Design review of the part built by this model. Coordinates are the model's own, in mm. A direction names the side the tool comes from. Coordinates: 2 decimals unless noted, no trailing zeros. Loops run counter-clockwise (first coordinate to the right, second up) from the corner with the lowest first, then second, coordinate; pieces in that order, holes last. Notation, with made-up numbers: (62.5, 24.25) -> (97.5, 24.25) arc R20 cw to (97.5, 41.25) -> close; hole circle Ø4 at (19, 31.5). An arc over 180 degrees is marked (long way). One line per item, written item: value. Start each with the question number.
1. Insertion check: pin 1 (8.5 mm diameter, centred on y = 10.75, z = -22.81, fed in from +X); pin 2 (5 mm diameter, centred on x = -26, y = 7.5, fed in from -Z); pin 3 (0.8 mm diameter, centred on x = 35, y = -48, fed in from -Z); pin 4 (0.8 mm diameter, centred on x = 35, y = 10.5, fed in from +Z). Each pin has a flat end and moves straight along its axis. Give the tip position at first contact, or say it passes through.
2. Add section B-B on z = -6. Write out the cut boundary in (x, y), plus the area to 3 significant figures.
3. Add section C-C on y = 41. Write out the cut boundary in (x, z), plus the area to 3 significant figures.
4. Add section A-A on x = 25. Write out the cut boundary in (y, z).
5. Draft analysis for pull direction X (two halves, no side actions). For faces 4 (the flat face through (34.5, -1, -53)), 5 (the flat face through (35.5, -1, -53)), 6 (the cylindrical face through (-35.007, -60.12, -8.277)), state which applies: pulls with the +X half, pulls with the -X half, needs draft (parallel to the pull), parting line crosses it, or undercut.
6. For probe 1 along X at (y, z) = (-39.5, -15); probe 2 along X at (y, z) = (-25, -29); probe 3 along Z at (x, y) = (-17, -59), list the stretches that pass through material, from the lowest coordinate up.
7. Machinability: for faces 1 (the cylindrical face through (-35.007, -59.896, -40.095)), 2 (the flat face through (-28, -5, -1)), 3 (the cylindrical face through (-35.007, 11.24, -26.555)), which of the approach directions +Z, -Z, +X, -X, +Y, -Y give a long, thin tool a straight path to every point of the face, cutting with its end or side? Answer none if there is none.
8. Add section D-D on y = 25. Write out the cut boundary in (x, z), plus the area to 3 significant figures.
```python
from build123d import *

# Parameters (mm, degrees)
BASE_FLANGE1_START             = -1
BASE_FLANGE1_OUTLINE_W         = 71
BASE_FLANGE1_OUTLINE_H         = 146.600550732
BASE_FLANGE1_DEPTH             = 1
EDGE_FLANGE1_STRIP_W           = 5.4732
EDGE_FLANGE1_STRIP_H           = 1
EDGE_FLANGE1_STRIP_CUT_DEPTH   = 146.600550732
EDGE_FLANGE1_STRIP_2_W         = 5.4732
EDGE_FLANGE1_STRIP_2_H         = 1
EDGE_FLANGE1_STRIP_CUT_2_DEPTH = 146.600550732
EDGE_FLANGE1_DEPTH             = 146.600550732
EDGE_FLANGE1_PROFILE_W         = 56.545302405
EDGE_FLANGE1_PROFILE_H         = 38.800406569
EDGE_FLANGE1_FLAT_DEPTH        = 1
EDGE_FLANGE1_BEND_DEPTH        = 146.600550732
EDGE_FLANGE1_PROFILE_2_W       = 146.600550732
EDGE_FLANGE1_PROFILE_2_H       = 72.095455735
EDGE_FLANGE1_PROFILE_2_R       = 3.775798506
EDGE_FLANGE1_PROFILE_2_R_2     = 3.613625218
EDGE_FLANGE1_FLAT_2_DEPTH      = 1


# Read off the part's stored shape, not the designer's step: Base-Flange1
# Sheet-metal steps are written as plain solids
with BuildPart() as part:
    # Base-Flange1 outline → Base-Flange1 (new body)
    with BuildSketch(Plane.XY.offset(BASE_FLANGE1_START)):
        Rectangle(BASE_FLANGE1_OUTLINE_W, BASE_FLANGE1_OUTLINE_H)
        Polygon((27.5, 56.679661992), (27.5, 35.987332772), (30.5, 35.987332772), (30.5, 3.276208649), (27.5, 3.276208649), (27.5, -51.054712488), (-27.5, -51.054712488), (-27.5, 3.276208649), (-30.5, 3.276208649), (-30.5, 35.987332772), (-27.5, 35.987332772), (-27.5, 56.679661992), align=None, mode=Mode.SUBTRACT)
    extrude(amount=BASE_FLANGE1_DEPTH)

    # Edge-Flange1 strip (across the edge) → Edge-Flange1 strip cut (cut)
    with BuildSketch(Plane(origin=(35.5, 73.300275366, -1), x_dir=(-1, 0, 0), z_dir=(0, -1, 0))):
        with Locations((-1, -0.5)):
            Rectangle(EDGE_FLANGE1_STRIP_W, EDGE_FLANGE1_STRIP_H)
    extrude(amount=EDGE_FLANGE1_STRIP_CUT_DEPTH, mode=Mode.SUBTRACT)

    # Edge-Flange1 strip 2 (across the edge) → Edge-Flange1 strip cut 2 (cut)
    with BuildSketch(Plane(origin=(-35.5, -73.300275366, -1), x_dir=(1, 0, 0), z_dir=(0, 1, 0))):
        with Locations((-1, -0.5)):
            Rectangle(EDGE_FLANGE1_STRIP_2_W, EDGE_FLANGE1_STRIP_2_H)
    extrude(amount=EDGE_FLANGE1_STRIP_CUT_2_DEPTH, mode=Mode.SUBTRACT)

    # Edge-Flange1 bend section (across the edge) → Edge-Flange1 (add)
    with BuildSketch(Plane(origin=(35.5, 73.300275366, -1), x_dir=(-1, 0, 0), z_dir=(0, -1, 0))):
        with BuildLine():
            Line((0, 0.7366), (1, 0.7366))
            ThreePointArc((1, 0.7366), (1.215745145, 0.215745145), (1.7366, 0))
            Line((1.7366, 0), (1.7366, -1))
            ThreePointArc((1.7366, -1), (0.508638364, -0.491361636), (0, 0.7366))
        make_face()
    extrude(amount=EDGE_FLANGE1_DEPTH)

    # Edge-Flange1 profile (on flange) → Edge-Flange1 flat (add)
    with BuildSketch(Plane(origin=(35.5, 0, -1), x_dir=(0, 1, 0), z_dir=(-1, 0, 0))):
        Polygon((-20.385230208, 70.874104098), (-20.385230208, 64.088111139), (-32.965566809, 64.088111139), (-32.965566809, 70.874104098), (-73.300275366, 70.874104098), (-73.300275366, 0.7366), (73.300275366, 0.7366), (73.300275366, 70.874104098), (29.936116194, 70.874104098), (29.936116194, 64.088111139), (14.177589294, 64.088111139), (14.177589294, 70.874104098), align=None)
        with Locations((0.339219033, 27.20786121)):
            Rectangle(EDGE_FLANGE1_PROFILE_W, EDGE_FLANGE1_PROFILE_H, mode=Mode.SUBTRACT)
    extrude(amount=EDGE_FLANGE1_FLAT_DEPTH)

    # Edge-Flange1 bend section 2 (across the edge) → Edge-Flange1 bend (add)
    with BuildSketch(Plane(origin=(-35.5, -73.300275366, -1), x_dir=(1, 0, 0), z_dir=(0, 1, 0))):
        with BuildLine():
            Line((0, 0.7366), (1, 0.7366))
            ThreePointArc((1, 0.7366), (1.215745145, 0.215745145), (1.7366, 0))
            Line((1.7366, 0), (1.7366, -1))
            ThreePointArc((1.7366, -1), (0.508638364, -0.491361636), (0, 0.7366))
        make_face()
    extrude(amount=EDGE_FLANGE1_BEND_DEPTH)

    # Edge-Flange1 profile 2 (on flange) → Edge-Flange1 flat 2 (add)
    with BuildSketch(Plane(origin=(-35.5, 0, -1), x_dir=(0, -1, 0), z_dir=(1, 0, 0))):
        with Locations((0, 36.784327868)):
            Rectangle(EDGE_FLANGE1_PROFILE_2_W, EDGE_FLANGE1_PROFILE_2_H)
        with BuildLine():
            ThreePointArc((65.114919352, 12.382584554), (60.007866854, 7.275532056), (54.900814356, 12.382584554))
            Line((54.900814356, 12.382584554), (54.900814356, 33.989345124))
            ThreePointArc((54.900814356, 33.989345124), (60.007866854, 39.096397622), (65.114919352, 33.989345124))
            Line((65.114919352, 33.989345124), (65.114919352, 12.382584554))
        make_face(mode=Mode.SUBTRACT)
        with Locations((-10.748889417, 21.810989166)):
            Circle(EDGE_FLANGE1_PROFILE_2_R, mode=Mode.SUBTRACT)
        with Locations((-10.748889417, 43.22132464)):
            Circle(EDGE_FLANGE1_PROFILE_2_R_2, mode=Mode.SUBTRACT)
    extrude(amount=EDGE_FLANGE1_FLAT_2_DEPTH)


solid = part.part
```
Worked answers:
1. pin 1: stops at x = -34.5
1. pin 2: passes through
1. pin 3: stops at z = -71.87
1. pin 4: stops at z = -0.21
2. outline: (-35.5, -73.3) -> (-34.5, -73.3) -> (-34.5, 73.3) -> (-35.5, 73.3) -> close; (34.5, -73.3) -> (35.5, -73.3) -> (35.5, 73.3) -> (34.5, 73.3) -> close
2. area: 293 mm²
3. outline: (-35.5, -73.83) -> (-34.5, -73.83) -> (-34.5, -1.74) arc R0.74 cw to (-33.76, -1) -> (-27.5, -1) -> (-27.5, 0) -> (-33.76, 0) arc R1.74 ccw to (-35.5, -1.74) -> close; (27.5, -1) -> (33.76, -1) arc R0.74 cw to (34.5, -1.74) -> (34.5, -71.87) -> (35.5, -71.87) -> (35.5, -1.74) arc R1.74 ccw to (33.76, 0) -> (27.5, 0) -> close
3. area: 159 mm²
4. outline: (-73.3, -1) -> (-51.05, -1) -> (-51.05, 0) -> (-73.3, 0) -> close; (56.68, -1) -> (73.3, -1) -> (73.3, 0) -> (56.68, 0) -> close
5. face 4: undercut
5. face 5: pulls with the +X half
5. face 6: needs draft
6. probe 1: x = -35.5 to -34.5, 34.5 to 35.5
6. probe 2: x = -35.5 to -34.5
6. probe 3: z = -1 to 0
7. face 1: -X
7. face 2: -Z, +Y, -Y
7. face 3: +X, -X
8. outline: (-35.5, -73.83) -> (-34.5, -73.83) -> (-34.5, -1.74) arc R0.74 cw to (-33.76, -1) -> (-30.5, -1) -> (-30.5, 0) -> (-33.76, 0) arc R1.74 ccw to (-35.5, -1.74) -> close; (30.5, -1) -> (33.76, -1) arc R0.74 cw to (34.5, -1.74) -> (34.5, -8.81) -> (35.5, -8.81) -> (35.5, -1.74) arc R1.74 ccw to (33.76, 0) -> (30.5, 0) -> close; (34.5, -65.09) -> (35.5, -65.09) -> (35.5, -47.61) -> (34.5, -47.61) -> close
8. area: 107 mm²
